Read the model definition and answer for the solid it produces. Units are mm, in the model's axes. Face numbers are marked on the shaded views. A direction names the side the tool comes from. Coordinates: 2 decimals unless noted, no trailing zeros. Order: outer loops, then holes, each group sorted by start corner. A loop starts at its lowest first (then second) coordinate and runs counter-clockwise, first axis right, second up. Notation, with made-up numbers: M -3,25.25 L 2,25.25 A30 ccw 2,50.25 Z; hole C 18,69.25 d9. An arc over 180 degrees is marked long. Put each result on its own line as item: value.
from build123d import *

# Parameters (mm, degrees)
BOTTOMBASES_R     = 1
BOTTOM_BASE_DEPTH = 4
MAINBASES_R       = 2.5
MAIN_BASE_DEPTH   = 0.5
WALLS_R           = 2.5
WALLS_R_2         = 2
WALL_DEPTH        = 1.5


with BuildPart() as part:
    # BottomBaseS → BOTTOM BASE (new body)
    with BuildSketch(Plane(origin=(0, 0, 0), x_dir=(1, 0, 0), z_dir=(0, 1, 0))):
        with Locations(Location((0, 0, 0), (0, 0, 270))):
            Circle(BOTTOMBASES_R)
    extrude(amount=-BOTTOM_BASE_DEPTH)

    # MainBaseS → MAIN BASE (add)
    with BuildSketch(Plane(origin=(0, 0, 0), x_dir=(1, 0, 0), z_dir=(0, 1, 0))):
        with Locations(Location((0, 0, 0), (0, 0, 270))):
            Circle(MAINBASES_R)
    extrude(amount=MAIN_BASE_DEPTH)

    # WallS → WALL (add)
    with BuildSketch(Plane(origin=(0, 0.5, 0), x_dir=(1, 0, 0), z_dir=(0, 1, 0))):
        with Locations(Location((0, 0, 0), (0, 0, 270))):
            Circle(WALLS_R)
        with Locations(Location((0, 0, 0), (0, 0, 270))):
            Circle(WALLS_R_2, mode=Mode.SUBTRACT)
    extrude(amount=WALL_DEPTH)


solid = part.part
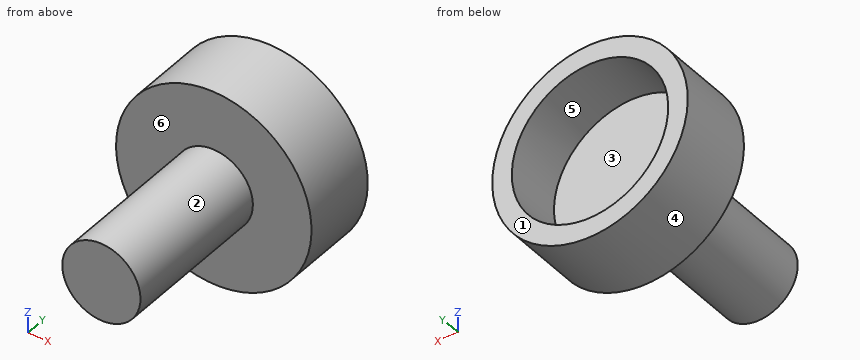
Q1. Find section B-B on x = 0. Write down the section's boundary in (y, z), plus the area to 3 significant figures.
Answers below:
outline: M -4,-1 L 0,-1 L 0,-2.5 L 2,-2.5 L 2,-2 L 0.5,-2 L 0.5,2 L 2,2 L 2,2.5 L 0,2.5 L 0,1 L -4,1 Z
area: 12.0 mm^2
Q2. Find section D-D on y = -1.5. Write down the section's boundary in (x, z), plus the area to 3 significant figures.
Answers below:
outline: C 0,0 d2
area: 3.14 mm^2
Q3. Consider line 1 along X through (y, z) = (1.45, 0); line 2 along Y through (x, z) = (0.7, -0.95); line 3 along Y through (x, z) = (-1.7, 1.3). Determine where each line is inside the solid, lowest interval first.
Answers below:
line 1: x = -2.5 to -2, 2 to 2.5
line 2: y = 0 to 0.5
line 3: y = 0 to 2
Q4. Given pin 1 (3 mm diameter, centred on y = -3, z = 1.5, fed in from +X); pin 2 (3 mm diameter, centred on x = -1, y = -3, fed in from +Z), each flat-ended and moving along its own axis, determine where each tip first touches the part or whether it passes through.
Answers below:
pin 1: stops at x = 1
pin 2: stops at z = 1
Q5. Find section C-C on y = 0.65. Write down the section's boundary in (x, z), plus the area to 3 significant figures.
Answers below:
outline: C 0,0 d5; hole C 0,0 d4
area: 7.07 mm^2
Q6. Find section A-A on z = 0. Write down the section's boundary in (x, y).
Answers below:
outline: M -2.5,0 L -1,0 L -1,-4 L 1,-4 L 1,0 L 2.5,0 L 2.5,2 L 2,2 L 2,0.5 L -2,0.5 L -2,2 L -2.5,2 Z
Q7. For a pull along X with two mould halves and no side action, classify the marked faces 1, 2 and 3 as +X half, -X half, draft (parallel to the pull), parting line (faces both ways), or undercut.
Answers below:
face 1: draft
face 2: parting line
face 3: undercut
Q8. A tool of negligible diameter and unlimited length cuts with its end or side. For the marked faces 4, 5 and 6, from which of +Z, -Z, +X, -X, +Y, -Y can it reach the whole face along a straight path? Write none if from no direction.
Answers below:
face 4: +Y, -Y
face 5: +Y
face 6: -Y
